```python
from build123d import *

# Parameters (mm, degrees)
SKETCH1_R                   = 1.5
BOSS_EXTRUDE1_DEPTH         = 6
FILLET1_R                   = 2
TAP_DRILL_FOR_M3_TAP1_D     = 2.5
TAP_DRILL_FOR_M3_TAP1_DEPTH = 10
TAP_DRILL_FOR_M3_TAP1_TIP   = 0.751075774


with BuildPart() as part:
    # Sketch1 → Boss-Extrude1 (new body)
    with BuildSketch(Plane(origin=(0, 0, 0), x_dir=(0, 0, -1), z_dir=(1, 0, 0))):
        Polygon((0, 0), (0, 15), (49.854455432, 52.772847367), (38.110170638, 81.126058999), (82.834388097, 99.651436437), (88.330517158, 86.382607119), (118.575687602, 98.910566914), (136.428533447, 55.809984346), (166.824723678, 43.219470108), (148.922633001, 0), (120, 0), (120, 5), (103.100505063, 12), (36.899494937, 12), (20, 5), (20, 0), align=None)
        with Locations((80, 60)):
            Circle(SKETCH1_R, mode=Mode.SUBTRACT)
        with Locations((125, 22)):
            Circle(SKETCH1_R, mode=Mode.SUBTRACT)
        with BuildLine():
            ThreePointArc((106.5, 60), (104.901854451, 69.063533798), (100.300177743, 77.033871657))
            ThreePointArc((100.300177743, 77.033871657), (98.186929663, 77.218756907), (98.002044413, 75.105508828))
            ThreePointArc((98.002044413, 75.105508828), (102.082776588, 68.037473368), (103.5, 60))
            ThreePointArc((103.5, 60), (105, 58.5), (106.5, 60))
        make_face(mode=Mode.SUBTRACT)
        with BuildLine():
            ThreePointArc((104.699822257, 39.033871657), (100.098145549, 31.063533798), (98.5, 22))
            ThreePointArc((98.5, 22), (100, 20.5), (101.5, 22))
            ThreePointArc((101.5, 22), (102.917223412, 30.037473368), (106.997955587, 37.105508828))
            ThreePointArc((106.997955587, 37.105508828), (106.813070337, 39.218756907), (104.699822257, 39.033871657))
        make_face(mode=Mode.SUBTRACT)
    extrude(amount=BOSS_EXTRUDE1_DEPTH)

    # Fillet1
    fillet1_edges = [part.edges().sort_by_distance(p)[0] for p in [
        (3, 15, 0),
        (3, 52.772847367, -49.854455432),
        (3, 81.126058999, -38.110170638),
        (3, 99.651436437, -82.834388097),
        (3, 86.382607119, -88.330517158),
        (3, 98.910566914, -118.575687602),
        (3, 55.809984346, -136.428533447),
        (3, 43.219470108, -166.824723678),
        (3, 5, -120),
        (3, 12, -103.100505063),
        (3, 12, -36.899494937),
        (3, 5, -20),
    ]]
    fillet(fillet1_edges, radius=FILLET1_R)

    # Tap Drill for M3 Tap1
    with Locations(Plane(origin=(0, 0, 0), x_dir=(-1, 0, 0), z_dir=(0, -1, 0))):
        with Locations((-3, 10), (-3, 130)):
            Hole(TAP_DRILL_FOR_M3_TAP1_D / 2, depth=TAP_DRILL_FOR_M3_TAP1_DEPTH)
            with Locations((0, 0, -(TAP_DRILL_FOR_M3_TAP1_DEPTH + TAP_DRILL_FOR_M3_TAP1_TIP / 2))):  # 118° drill point
                Cone(0, TAP_DRILL_FOR_M3_TAP1_D / 2, TAP_DRILL_FOR_M3_TAP1_TIP, mode=Mode.SUBTRACT)


solid = part.part
```
Part model, mm, in its own coordinate system. A direction names the side the tool comes from. Round coordinates to 2 decimals unless told otherwise and drop trailing zeros. Order: outer loops, then holes, each group sorted by start corner. A loop starts at its lowest first (then second) coordinate and runs counter-clockwise, first axis right, second up. Notation, with made-up numbers: M 65,-16.75 L 82,-16.75 A21 ccw 82,-11.75 Z; hole C 60.25,75.25 d7. An arc over 180 degrees is marked long. Put each result on its own line as item: value. Start each with the question number.
1. Drill centre lines: probe 1 along X at (y, z) = (7, -10); probe 2 along Z at (x, y) = (3, 4.5); probe 3 along Z at (x, y) = (4, 95.5). Where is each one in solid material? Low to high. Write a range as [from, to].
2. Slice it at A-A on y = 66.5. List the corners of the cut face in (x, z), then the cut area to 3 significant figures.
3. Drop flat-ended pins along their axis: pin 1 (1 mm diameter, centred on x = 4.5, y = 70, fed in from -Z); pin 2 (1.5 mm diameter, centred on x = 4, y = 40, fed in from -Z); pin 3 (1.1 mm diameter, centred on x = 1.5, y = 1.5, fed in from -Z). Give the stop position or say it passes through.
4. Slice it at B-B on z = -76. List the corners of the cut face in (x, y).
5. Tool access for faces 4 (the face through (3, 12, -70)), 5 (the face through (3, 58.5, -105)), 6 (the face through (2.96, 92.57, -103.27)), 7 (the face through (2.958, 33.467, -24.373)): list every direction of +Z, -Z, +X, -X, +Y, -Y with a clear straight run to the whole face (end or side of a thin tool).
6. Two-plate mould, pull along Z, no slides. Class faces 1 (the face through (2.958, 8.724, -28.99)), 2 (the face through (6, 39, -84)), 3 (the face through (2.96, 77.1, -127.61)): +Z half, -Z half, draft (parallel to the pull), parting line (faces both ways), or undercut.
Findings:
1. probe 1: [0, 1.75], [4.25, 6]
1. probe 2: [-150.79, -131.25], [-128.75, -119.82], [-20.18, -11.25], [-8.75, 0]
1. probe 3: [-119.99, -110.34], [-84.55, -72.81]
2. outline: M 0,-132 L 6,-132 L 6,-105.69 L 0,-105.69 Z; M 0,-102.58 L 6,-102.58 L 6,-44.17 L 0,-44.17 Z
2. area: 508 mm2
3. pin 1: z = -130.76
3. pin 2: z = -165.8
3. pin 3: z = -149.77
4. outline: M 0,12 L 6,12 L 6,96.82 L 0,96.82 Z
5. face 4: +X, -X, -Y
5. face 5: +X, -X
5. face 6: +X, -X, +Y
5. face 7: +Z, +X, -X
6. face 1: undercut
6. face 2: draft
6. face 3: -Z half
